Could you check a few things on this model? Use its own coordinates, in mm. A direction names the side the tool comes from. Give positions to 0.01 mm unless a question says otherwise; leave off trailing zeros. Loops run counter-clockwise (first coordinate to the right, second up) from the corner with the lowest first, then second, coordinate; pieces in that order, holes last. Notation, with made-up numbers: M -2.5,11 L 28.5,11 A19 ccw 28.5,48 Z; hole C 69.25,18.25 d3. An arc over 180 degrees is marked long. Answer in a Markdown table with one row per item. Add a question column.
1. I need wall thicknesses on line 1 along Y through (x, z) = (12.5, -10); line 2 along Y through (x, z) = (-11, 1); line 3 along Y through (x, z) = (8, 15). Which ranges of each line are inside material? Lowest first, please. Write a range as from..to.
2. Thinking about a two-plate mould opening in Y: for faces 5 (the cylindrical face through (13.17, 10.47, 9.01)), 6 (the conical face through (17.58, 38.506, 5.536)), 7 (the flat face through (-19, 11.2, -8)), which applies, released by +Y, released by -Y, zero draft, split by the parting line, or undercut?
3. If we section it at B-B on y = 37.5: List the corners of the cut face in (x, z) for me, then the cut area to 3 significant figures.
4. If we section it at A-A on y = 9.5: List the corners of the cut face in (x, z) for me, then the cut area to 3 significant figures.
5. I'm going to push flat-ended pins straight in: pin 1 Ø2 at (x, z) = (-8.5, 5.5) entering from +Y; pin 2 Ø6 at (x, z) = (5.5, -9) entering from -Y; pin 3 Ø21 at (x, z) = (6.5, -6.5) entering from +Y; pin 4 Ø3 at (x, z) = (-9.37, 14.78) entering from -Y. Where does each tip first touch, or does it pass through?
6. Which directions (+Z, -Z, +X, -X, +Y, -Y) give clear straight access to the entire face, cutting with the end or side of a thin tool? Please do faces 1 (the cylindrical face through (3.233, 41.235, -1.341)), 2 (the cylindrical face through (-13.145, 16.242, -9.583)), 3 (the flat face through (-14, 16, 13)), 4 (the flat face through (-9, 13.2, 5)).
```python
from build123d import *

# Parameters (mm, degrees)
SKETCH_2_W             = 28
SKETCH_2_H             = 4.5
CUT_EXTRUDE_1_DEPTH    = 10
EXTRUDE_1_DEPTH        = 15
HOLE_WIZARD_M4_2_D     = 3.3
HOLE_WIZARD_M4_2_DEPTH = 10.5
HOLE_WIZARD_M4_2_TIP   = 0.991420021


with BuildPart() as part:
    # 草图1 → 旋转1 (revolve)
    with BuildSketch(Plane.XY):
        Polygon((0, 0), (4.1, 0), (4.1, 6.7), (13.4, 6.7), (13.4, 8.7), (21, 8.7), (21, 10.2), (20, 10.2), (20, 11.2), (21, 11.2), (21, 12.2), (10, 12.2), (10, 13.2), (21, 13.2), (21, 20.4), (5, 20.4), (5, 21), (21, 21), (21, 34.7), (18.3, 38.7), (3.5, 38.7), (3.5, 43.7), (0, 43.7), align=None)
    revolve(axis=Axis((0, 43.7, 0), (0, -1, 0)))

    # 草图2 → 切除-拉伸1 (cut)
    with BuildSketch(Plane.XY.offset(21)):
        with Locations((0, 16.05)):
            Rectangle(SKETCH_2_W, SKETCH_2_H)
    extrude(amount=-CUT_EXTRUDE_1_DEPTH, mode=Mode.SUBTRACT)

    # 草图3 → 凸台-拉伸1 (add)
    with BuildSketch(Plane.XY.offset(11)):
        with BuildLine():
            Line((9.185056323, 18.053194417), (9.385056323, 18.053194417))
            ThreePointArc((9.385056323, 18.053194417), (11.385056323, 16.053194417), (9.385056323, 14.053194417))
            Line((9.385056323, 14.053194417), (9.185056323, 14.053194417))
            ThreePointArc((9.185056323, 14.053194417), (7.185056323, 16.053194417), (9.185056323, 18.053194417))
        make_face()
    extrude(amount=EXTRUDE_1_DEPTH)

    # M4 螺纹孔2
    with Locations(Plane(origin=(-14.780985523, 8.7, -9.368696119), x_dir=(0, 0, -1), z_dir=(0, -1, 0))):
        with Locations((0, 0), (-24.149681642, 5.412289404), (5.412289404, 24.149681642), (-18.737392238, 29.561971046)):
            Hole(HOLE_WIZARD_M4_2_D / 2, depth=HOLE_WIZARD_M4_2_DEPTH)
            with Locations((0, 0, -(HOLE_WIZARD_M4_2_DEPTH + HOLE_WIZARD_M4_2_TIP / 2))):  # 118° drill point
                Cone(0, HOLE_WIZARD_M4_2_D / 2, HOLE_WIZARD_M4_2_TIP, mode=Mode.SUBTRACT)


solid = part.part
```
Results:
| question | item | result |
|---|---|---|
| 1 | line 1 | 8.7..12.2, 13.2..20.4, 21..38.7 |
| 1 | line 2 | 6.7..12.2, 13.2..20.4, 21..38.7 |
| 1 | line 3 | 8.7..12.2, 13.2..13.8, 14.44..17.66, 18.3..20.4, 21..38.7 |
| 2 | face 5 | zero draft |
| 2 | face 6 | released by +Y |
| 2 | face 7 | undercut |
| 3 | outline | C 0,0 d38.22 |
| 3 | area | 1,150 mm2 |
| 4 | outline | C 0,0 d42; hole C -14.78,-9.37 d3.3; hole C -9.37,14.78 d3.3; hole C 9.37,-14.78 d3.3; hole C 14.78,9.37 d3.3 |
| 4 | area | 1,350 mm2 |
| 5 | pin 1 | y = 38.7 |
| 5 | pin 2 | y = 6.7 |
| 5 | pin 3 | y = 43.7 |
| 5 | pin 4 | y = 19.29 |
| 6 | face 1 | +Y |
| 6 | face 2 | -Y |
| 6 | face 3 | +Z |
| 6 | face 4 | none |
